from build123d import *

# Parameters (mm, degrees)
MAKERBEAMFIX_DEPTH          = 22.5
SKETCH4_R                   = 1.5
FIXINGHOLE_DEPTH            = 16
SKETCH5_R                   = 4.25
DRIVERHOLE_DEPTH            = 12
HOLEFORCALIBERS_DEPTH       = 4.2
CUT_EXTRUDE2_DEPTH          = 16
SKETCH8_W                   = 12
SKETCH8_H                   = 2.8
CUT_EXTRUDE3_DEPTH          = 46
SKETCH9_W                   = 2
SKETCH9_H                   = 8
HOLEFORSCREWOFCALIBER_DEPTH = 49.643043085


with BuildPart() as part:
    # Sketch1 → MakerBeamFix (new body, symmetric)
    with BuildSketch(Plane.XY):
        Polygon((-11, 0), (11, 0), (11, 14), (7.45, 14), (7.45, 15), (4.55, 15), (4.55, 14), (-11, 14), align=None)
    extrude(amount=MAKERBEAMFIX_DEPTH, both=True)

    # Sketch4 → FixingHole (cut, through all)
    with BuildSketch(Plane.XZ):
        with Locations((6, 0)):
            Circle(SKETCH4_R)
    extrude(amount=-FIXINGHOLE_DEPTH, mode=Mode.SUBTRACT)

    # Sketch5 → DriverHole (cut, through all)
    with BuildSketch(Plane(origin=(0, 11, 0), x_dir=(1, 0, 0), z_dir=(0, 1, 0))):
        with Locations((6, 0)):
            Circle(SKETCH5_R)
    extrude(amount=-DRIVERHOLE_DEPTH, mode=Mode.SUBTRACT)

    # Sketch6 → HoleForCalibers (cut)
    with BuildSketch(Plane(origin=(0, 4, 0), x_dir=(1, 0, 0), z_dir=(0, 1, 0))):
        Polygon((7.420739047, -26.899923767), (-9, -22.5), (3.589745962, 24.485571585), (20.010485009, 20.085647818), align=None)
    extrude(amount=HOLEFORCALIBERS_DEPTH, mode=Mode.SUBTRACT)

    # Sketch7 → Cut-Extrude2 (cut, through all)
    with BuildSketch(Plane(origin=(0, 0, 0), x_dir=(-1, 0, 0), z_dir=(0, -1, 0))):
        Polygon((11, 22.5), (-1.057713659, 22.5), (11, -22.5), align=None)
    extrude(amount=-CUT_EXTRUDE2_DEPTH, mode=Mode.SUBTRACT)

    # Sketch8 → Cut-Extrude3 (cut, through all)
    with BuildSketch(Plane.XY.offset(22.5)):
        with Locations((-5, 12.6)):
            Rectangle(SKETCH8_W, SKETCH8_H)
    extrude(amount=-CUT_EXTRUDE3_DEPTH, mode=Mode.SUBTRACT)

    # Sketch9 → HoleForScrewOfCaliber (cut, through all)
    with BuildSketch(Plane(origin=(-6.227885683, 0, 23.242785793), x_dir=(0, -1, 0), z_dir=(-0.258819045, 0, 0.965925826))):
        with Locations((-3, 1.130096078)):
            Rectangle(SKETCH9_W, SKETCH9_H)
    extrude(amount=-HOLEFORSCREWOFCALIBER_DEPTH, mode=Mode.SUBTRACT)


solid = part.part
Input: part model. Units: mm. Frame: model coordinates. A direction names the side the tool comes from. Give positions to 0.01 mm unless a question says otherwise; leave off trailing zeros. Order: outer loops, then holes, each group sorted by start corner. A loop starts at its lowest first (then second) coordinate and runs counter-clockwise, first axis right, second up. Notation, with made-up numbers: (33, 1) - (72, 1) arc R10 cw to (72, 14) - close; hole circle Ø1 at (27, 55). An arc over 180 degrees is marked (long way). Answer as a JSON object with one key per item and string values. Group by question number.
Q1. Cut plane D-D, the plane y = 1.5. Output: boundary loops of the cut face in (x, z).
Q2. First-contact query: pin 1 Ø6 at (y, z) = (7.5, -10) entering from -X; pin 2 Ø0.5 at (y, z) = (14.5, 9.5) entering from -X; pin 3 Ø1.1 at (y, z) = (14.5, -16) entering from -X. Flat tips, straight axial feed; report the tip coordinate or a pass-through.
Q3. Cut plane A-A, the plane y = 5.25. Output: boundary loops of the cut face in (x, z).
Q4. Line query: probe 1 along Z at (x, y) = (6, 8.85); probe 2 along Y at (x, z) = (3, 10); probe 3 along Y at (x, z) = (-5.75, 20). Output: solid intervals per line, ascending.
Q5. Set-up query: faces 1 (the face through (-2, 11.2, 10)), 2 (the face through (1.74, 3.01, 13.32)), 3 (the face through (8, 11, 0)), 4 (the face through (-4.89, 5.35, -0.31)), 5 (the face through (7.45, 14.5, -11.3)). Return all of +Z, -Z, +X, -X, +Y, -Y with unobstructed straight access to the full face (end or side cutting, diameter ignored); none if empty.
Q6. Mould query, pull axis Z, two halves, no side actions, for faces 6 (the face through (8.69, 3.01, -12.61)), 7 (the face through (1, 13, 0)), 8 (the face through (7.386, 12.972, -0.575)). Classes: pulls with the +Z half, pulls with the -Z half, needs draft (parallel to the pull), parting line crosses it, or undercut.
Q7. Cut plane C-C, the plane z = 16. Output: boundary loops of the cut face in (x, y).
Q8. Cut plane B-B, the plane x = 6. Output: boundary loops of the cut face in (y, z), then the cut area to 3 significant figures.
Results:
{
 "1": {"outline": "(-11, 22.5) - (1.06, -22.5) - (11, -22.5) - (11, 22.5) - close; hole circle Ø8.5 at (6, 0)"},
 "2": {"pin 1": "x = -3.1", "pin 2": "x = 4.55", "pin 3": "x = 1"},
 "3": {"outline": "(-11, 22.5) - (1.06, -22.5) - (3.06, -22.5) - (-9, 22.5) - close; (8.6, 22.5) - (11, 13.54) - (11, 22.5) - close"},
 "4": {"probe 1": "-22.5 to -4.25, 4.25 to 22.5", "probe 2": "0 to 4, 8.2 to 14", "probe 3": "0 to 2, 8.2 to 11.2"},
 "5": {"face 1": "+Z, -Z, -X, +Y", "face 2": "none", "face 3": "-Y", "face 4": "-Z, -X, +Y, -Y", "face 5": "+Z, -Z, +X, +Y"},
 "6": {"face 6": "pulls with the -Z half", "face 7": "needs draft", "face 8": "undercut"},
 "7": {"outline": "(-9.26, 0) - (11, 0) - (11, 14) - (7.45, 14) - (7.45, 15) - (4.55, 15) - (4.55, 14) - (1, 14) - (1, 11.2) - (-9.26, 11.2) - close; hole (-7.26, 2) - (1.02, 2) - (1.02, 4) - (10.34, 4) - (10.34, 8.2) - (-7.26, 8.2) - close"},
 "8": {"outline": "(0, -22.5) - (2, -22.5) - (2, -4.25) - (0, -4.25) - close; (0, 4.25) - (4, 4.25) - (4, 22.5) - (0, 22.5) - close; (8.2, -22.5) - (15, -22.5) - (15, -1.5) - (11, -1.5) - (11, -4.25) - (8.2, -4.25) - close; (8.2, 4.25) - (11, 4.25) - (11, 1.5) - (15, 1.5) - (15, 22.5) - (8.2, 22.5) - close", "area": "380 mm^2"}
}
